Part model, mm, in its own coordinate system. Give positions to 0.01 mm unless a question says otherwise; leave off trailing zeros. Write each loop counter-clockwise with the first axis right and the second up, starting at its lowest first coordinate (ties: lowest second). Pieces come first, ordered by that corner, then holes. Notation, with made-up numbers: M 88,76 L 106,76 A19 cw 106,83 Z; hole C 21.25,60.25 d5. An arc over 180 degrees is marked long. Use CSV: the item, a comma, the result in double quotes. Start each with the question number.
1. Drill centre lines: line 1 along Y through (x, z) = (27.8, 27.3); line 2 along Y through (x, z) = (27, 27). Where is each one in solid material? Low to high. Write a range as from..to.
2. Drop a flat-ended pin along its axis: pin 1 Ø5 at (x, y) = (27.8, 10) entering from +Z. Give the stop position or say it passes through.
3. Band-saw the part on A-A, the plane x = 27.8. List the corners of the cut face in (y, z), then the cut area to 3 significant figures.
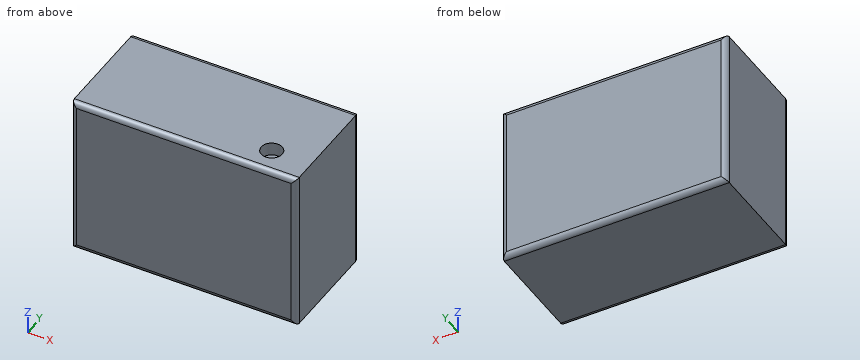
from build123d import *

# Parameters (mm, degrees)
SKETCH_1_W          = 85.6
SKETCH_1_H          = 61.6
EXTRUDE_1_DEPTH     = 42
SKETCH_2_R          = 4
CUT_EXTRUDE_1_DEPTH = 5
FILLET_1_R          = 2


with BuildPart() as part:
    # 草图1 → 凸台-拉伸1 (new body)
    with BuildSketch(Plane(origin=(0, 0, 0), x_dir=(1, 0, 0), z_dir=(0, 1, 0))):
        Rectangle(SKETCH_1_W, SKETCH_1_H)
    extrude(amount=EXTRUDE_1_DEPTH)

    # 草图2 → 切除-拉伸1 (cut)
    with BuildSketch(Plane.XY.offset(30.8)):
        with Locations((27.8, 10)):
            Circle(SKETCH_2_R)
    extrude(amount=-CUT_EXTRUDE_1_DEPTH, mode=Mode.SUBTRACT)

    # 圆角1
    fillet_1_edges = [part.edges().sort_by_distance(p)[0] for p in [
        (-42.8, 42, 0),
        (0, 42, 30.8),
        (42.8, 42, 0),
        (0, 0, 30.8),
        (-42.8, 0, 0),
        (0, 0, -30.8),
        (42.8, 0, 0),
        (0, 42, -30.8),
    ]]
    fillet(fillet_1_edges, radius=FILLET_1_R)


solid = part.part
Output:
1,line 1,"y = 0..6, 14..42"
1,line 2,"y = 0..6.08, 13.92..42"
2,pin 1,"stops at z = 25.8"
3,outline,"M 0,-28.8 A2 ccw 2,-30.8 L 40,-30.8 A2 ccw 42,-28.8 L 42,28.8 A2 ccw 40,30.8 L 14,30.8 L 14,25.8 L 6,25.8 L 6,30.8 L 2,30.8 A2 ccw 0,28.8 Z"
3,area,"2,540 mm²"
